CAD build for the part. Positions are in the model's coordinates, mm. A direction names the side the tool comes from. Round coordinates to 2 decimals unless told otherwise and drop trailing zeros. Loops run counter-clockwise (first coordinate to the right, second up) from the corner with the lowest first, then second, coordinate; pieces in that order, holes last.
Autodesk Inventor part; units mm, degrees
ref_plane "YZ Plane" through (0, 0, 0) normal (1, 0, 0) x (0, 1, 0)
ref_plane "XZ Plane" through (0, 0, 0) normal (0, 1, 0) x (-1, 0, 0)
ref_plane "XY Plane" through (0, 0, 0) normal (0, 0, 1) x (1, 0, 0)
sketch "Sketch1" plane through (0, 0, 0) normal (0, 1, 0) x (-1, 0, 0)
  line L0 (0, 0) -> (80, 0)
  line L1 (80, 0) -> (80, 20)
  line L2 (80, 20) -> (0, 20)
  line L3 (0, 20) -> (0, 0)
  circle A0 centre (65, 10) radius 2.6
  dimension "d2" = 20
  dimension "d3" = 80
  dimension "d4" = 5.2
  dimension "d7" = 15
  dimension "d8" = 10
extrude "Extrusion2" add sketch "Sketch1" along normal blind 5
sketch "Sketch3" plane through (0, 5, 0) normal (0, 1, 0) x (1, 0, 0)
  circle A0 centre (-65, -10) radius 2.6
  line L0 (0, 0) -> (-80, 0)
  line L1 (-80, 0) -> (-80, -20)
  line L2 (-80, -20) -> (0, -20)
  line L3 (0, -20) -> (0, 0)
  line L4 (-10.5, -5) -> (-20.5, -5)
  line L5 (-20.5, -5) -> (-20.5, -15)
  line L6 (-20.5, -15) -> (-10.5, -15)
  line L7 (-10.5, -15) -> (-10.5, -5)
  line L8 (-10.5, -5) -> (-20.5, -15) construction
  line L9 (-20.5, -5) -> (-10.5, -15) construction
  point P0 (-15.5, -10)
  dimension "d11" = 10
  dimension "d12" = 10
  dimension "d17" = 64.5
  dimension "d18" = 10
extrude "Extrusion3" cut sketch "Sketch3" against normal through all contours L7 L6 L5 L4
equation "\"d8\" = 0.5 * d2"
properties part number "slider_box" material "Wood (Birch)"
Item 1: Cut at C-C, the plane y = 3.55. Give the cut face in (x, z).
Answers follow:
outline: (-80, 0) - (0, 0) - (0, 20) - (-80, 20) - close; hole circle Ø5.2 at (-65, 10); hole (-20.5, 5) - (-10.5, 5) - (-10.5, 15) - (-20.5, 15) - close
Item 2: Cut at A-A, the plane z = 9. Give the cut face in (x, y).
Answers follow:
outline: (-80, 0) - (-67.4, 0) - (-67.4, 5) - (-80, 5) - close; (-62.6, 0) - (-20.5, 0) - (-20.5, 5) - (-62.6, 5) - close; (-10.5, 0) - (0, 0) - (0, 5) - (-10.5, 5) - close
Item 3: 3-axis set-ups, long thin cutter, end or side, ignore diameter. For faces 4 (the flat face through (-15, 3, 5)), 5 (the flat face through (-41, 2, 20)): which of +Z, -Z, +X, -X, +Y, -Y reach the whole face in a straight line?
Answers follow:
face 4: +Y, -Y
face 5: +Z, +X, -X, +Y, -Y
Item 4: Two-plate mould, pull along Z, no slides. Class faces 1 (the flat face through (-39, 5, 10)), 2 (the flat face through (-10.5, 3, 10)), 3 (the flat face through (-39, 2, 0)): released by +Z, released by -Z, zero draft, split by the parting line, or undercut.
Answers follow:
face 1: zero draft
face 2: undercut
face 3: released by -Z
Item 5: Cut at D-D, the plane x = -65. Give the cut face in (y, z), plus the area to 3 significant figures.
Answers follow:
outline: (0, 0) - (5, 0) - (5, 7.4) - (0, 7.4) - close; (0, 12.6) - (5, 12.6) - (5, 20) - (0, 20) - close
area: 74.0 mm2
Item 6: Cut at B-B, the plane z = 13.75. Give the cut face in (x, y).
Answers follow:
outline: (-80, 0) - (-20.5, 0) - (-20.5, 5) - (-80, 5) - close; (-10.5, 0) - (0, 0) - (0, 5) - (-10.5, 5) - close
Item 7: Probe line 1 (Z direction, x = -16, y = 0.65); line 2 (X direction, y = 4.2, z = 6); line 3 (X direction, y = 4.2, z = 11.75). List the from-to ranges inside material, lowest first.
Answers follow:
line 1: z = 0 to 5, 15 to 20
line 2: x = -80 to -20.5, -10.5 to 0
line 3: x = -80 to -66.92, -63.08 to -20.5, -10.5 to 0
